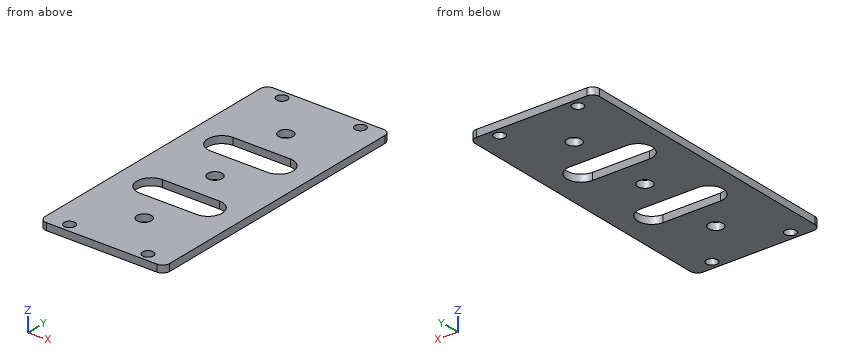
from build123d import *

# Parameters (mm, degrees)
SKETCH_1_W               = 35
SKETCH_1_H               = 80
EXTRUDE_1_DEPTH          = 2
SKETCH_2_R               = 1.525
CUT_EXTRUDE_1_DEPTH      = 2
FILLET_1_R               = 2
SKETCH_3_R               = 2.025
CUT_EXTRUDE_2_DEPTH      = 10
CUT_EXTRUDE_3_DEPTH      = 1
CUT_EXTRUDE_3_DEPTH_BACK = 3


with BuildPart() as part:
    # 草图1 → 凸台-拉伸1 (new body)
    with BuildSketch(Plane.XY):
        Rectangle(SKETCH_1_W, SKETCH_1_H)
    extrude(amount=EXTRUDE_1_DEPTH)

    # 草图2 → 切除-拉伸1 (cut)
    with BuildSketch(Plane.XY.offset(2)):
        with Locations((11, 37.5)):
            Circle(SKETCH_2_R)
        with Locations((-11, 37.5)):
            Circle(SKETCH_2_R)
        with Locations((-11, -37.5)):
            Circle(SKETCH_2_R)
        with Locations((11, -37.5)):
            Circle(SKETCH_2_R)
    extrude(amount=-CUT_EXTRUDE_1_DEPTH, mode=Mode.SUBTRACT)

    # 圆角1
    fillet_1_edges = [part.edges().sort_by_distance(p)[0] for p in [
        (17.5, -40, 1),
        (-17.5, -40, 1),
        (-17.5, 40, 1),
        (17.5, 40, 1),
    ]]
    fillet(fillet_1_edges, radius=FILLET_1_R)

    # 草图3 → 切除-拉伸2 (cut)
    with BuildSketch(Plane.XY.offset(2)):
        with Locations((0, 25)):
            Circle(SKETCH_3_R)
        Circle(SKETCH_3_R)
        with Locations((0, -25)):
            Circle(SKETCH_3_R)
    extrude(amount=-CUT_EXTRUDE_2_DEPTH, mode=Mode.SUBTRACT)

    # 草图4 → 切除-拉伸3 (cut, two sides)
    with BuildSketch(Plane.XY.offset(2)) as cut_extrude_3_sk:
        with BuildLine():
            Line((-8, 16.5), (8, 16.5))
            ThreePointArc((8, 16.5), (12, 12.5), (8, 8.5))
            Line((8, 8.5), (-8, 8.5))
            ThreePointArc((-8, 8.5), (-12, 12.5), (-8, 16.5))
        make_face()
        with BuildLine():
            Line((-8, -16.5), (8, -16.5))
            ThreePointArc((8, -16.5), (12, -12.5), (8, -8.5))
            Line((8, -8.5), (-8, -8.5))
            ThreePointArc((-8, -8.5), (-12, -12.5), (-8, -16.5))
        make_face()
    extrude(amount=CUT_EXTRUDE_3_DEPTH, mode=Mode.SUBTRACT)
    extrude(cut_extrude_3_sk.sketch, amount=-CUT_EXTRUDE_3_DEPTH_BACK, mode=Mode.SUBTRACT)


solid = part.part
Model file for the job. Use its own axes, mm. Round coordinates to 2 decimals unless told otherwise and drop trailing zeros. Loops run counter-clockwise (first coordinate to the right, second up) from the corner with the lowest first, then second, coordinate; pieces in that order, holes last. Notation, with made-up numbers: M 32,-36 L 52,-36 A18 ccw 52,-28 Z; hole C 16.25,-11.5 d4. An arc over 180 degrees is marked long. One line per question, with ' | ' between items.
1) Band-saw the part on D-D (y = 0). Give the cut face in (x, z) (3 decimals).
Solved:
outline: M -17.5,0 L -2.025,0 L -2.025,2 L -17.5,2 Z; M 2.025,0 L 17.5,0 L 17.5,2 L 2.025,2 Z
2) Band-saw the part on C-C (x = -3). Give the cut face in (y, z), then the cut area to 3 significant figures.
Solved:
outline: M -40,0 L -16.5,0 L -16.5,2 L -40,2 Z; M -8.5,0 L 8.5,0 L 8.5,2 L -8.5,2 Z; M 16.5,0 L 40,0 L 40,2 L 16.5,2 Z | area: 128 mm²
3) Drill centre lines: line 1 along Y through (x, z) = (0, 0.4) (3 decimals); line 2 along Y through (x, z) = (8, 1.15); line 3 along Y through (x, z) = (11, 1.2) (3 decimals). Where is each one in solid material? Low to high.
Solved:
line 1: y = -40 to -27.025, -22.975 to -16.5, -8.5 to -2.025, 2.025 to 8.5, 16.5 to 22.975, 27.025 to 40 | line 2: y = -40 to -16.5, -8.5 to 8.5, 16.5 to 40 | line 3: y = -40 to -39.025, -35.975 to -15.146, -9.854 to 9.854, 15.146 to 35.975, 39.025 to 40
4) Band-saw the part on B-B (z = 0.85). Give the number of separate pieces and of enclosed holes in the cut face, then the cut area to 3 significant figures.
Solved:
separate pieces: 1 | enclosed holes: 9 | area: 2,370 mm²
5) Flat gauge pins, fed straight in: pin 1 (6 mm diameter, centred on x = 11, y = -4, fed in from -Z); pin 2 (3.5 mm diameter, centred on x = 0, y = 0, fed in from +Z). Where does each tip first touch, or does it go through?
Solved:
pin 1: stops at z = 0 | pin 2: passes through
6) Band-saw the part on A-A (y = 12.5). Give the cut face in (x, z).
Solved:
outline: M -17.5,0 L -12,0 L -12,2 L -17.5,2 Z; M 12,0 L 17.5,0 L 17.5,2 L 12,2 Z
